Work out the finished part from the listing and answer in its coordinate system (mm). A direction names the side the tool comes from. Round coordinates to 2 decimals unless told otherwise and drop trailing zeros. Loops run counter-clockwise (first coordinate to the right, second up) from the corner with the lowest first, then second, coordinate; pieces in that order, holes last.
from build123d import *

# Parameters (mm, degrees)
SKETCH_1_W           = 149
SKETCH_1_H           = 70
EXTRUDE_1_DEPTH      = 1
SKETCH_2_W           = 147
SKETCH_2_H           = 68
EXTRUDE_2_DEPTH      = 2
FILLET_1_R           = 5
SKETCH_3_W           = 3
SKETCH_3_H           = 26
EXTRUDE_3_DEPTH      = 10
FILLET_2_R           = 4
SKETCH_6_R           = 3.5
EXTRUDE_4_DEPTH      = 4
SKETCH_7_W           = 86.66
SKETCH_7_H           = 55.5
CUT_EXTRUDE_3_DEPTH  = 2
SKETCH_8_W           = 74
SKETCH_8_H           = 49
CUT_EXTRUDE_4_DEPTH  = 2
SKETCH_11_R          = 4
CUT_EXTRUDE_7_DEPTH  = 4
SKETCH_12_R          = 1.35
CUT_EXTRUDE_8_DEPTH  = 4
SKETCH_13_R          = 1.35
CUT_EXTRUDE_9_DEPTH  = 4
SKETCH_14_R          = 1.35
CUT_EXTRUDE_10_DEPTH = 4
SKETCH_15_W          = 14
SKETCH_15_H          = 13.5
CUT_EXTRUDE_11_DEPTH = 4
SKETCH_9_R           = 3.5
CUT_EXTRUDE_12_DEPTH = 4
SKETCH_16_R          = 3.5
CUT_EXTRUDE_13_DEPTH = 4
EXTRUDE_5_DEPTH      = 4
EXTRUDE_6_DEPTH      = 1


with BuildPart() as part:
    # Эскиз1 → Бобышка-Вытянуть1 (new body)
    with BuildSketch(Plane.XY):
        Rectangle(SKETCH_1_W, SKETCH_1_H)
    extrude(amount=EXTRUDE_1_DEPTH)

    # Эскиз2 → Бобышка-Вытянуть2 (add)
    with BuildSketch(Plane.XY.offset(1)):
        Rectangle(SKETCH_2_W, SKETCH_2_H)
    extrude(amount=EXTRUDE_2_DEPTH)

    # Скругление1
    fillet_1_edges = [part.edges().sort_by_distance(p)[0] for p in [
        (-73.5, 34, 2),
        (-73.5, -34, 2),
        (73.5, -34, 2),
        (73.5, 34, 2),
        (-74.5, 35, 0.5),
        (74.5, 35, 0.5),
        (74.5, -35, 0.5),
        (-74.5, -35, 0.5),
    ]]
    fillet(fillet_1_edges, radius=FILLET_1_R)

    # Эскиз3 → Бобышка-Вытянуть3 (add)
    with BuildSketch(Plane.XY.offset(3)):
        with Locations((-72, 1)):
            Rectangle(SKETCH_3_W, SKETCH_3_H)
        with Locations((72, 1)):
            Rectangle(SKETCH_3_W, SKETCH_3_H)
    extrude(amount=EXTRUDE_3_DEPTH)

    # Скругление2
    fillet_2_edges = [part.edges().sort_by_distance(p)[0] for p in [
        (-72, -12, 13),
        (-72, 14, 13),
        (72, 14, 13),
        (72, -12, 13),
    ]]
    fillet(fillet_2_edges, radius=FILLET_2_R)

    # Эскиз6 → Бобышка-Вытянуть4 (add)
    with BuildSketch(Plane.XY.offset(3)):
        with Locations((-67.16, 29.285)):
            Circle(SKETCH_6_R)
        with Locations((67.16, 29.285)):
            Circle(SKETCH_6_R)
        with Locations((-67.16, -29.285)):
            Circle(SKETCH_6_R)
    extrude(amount=EXTRUDE_4_DEPTH)

    # Эскиз7 → Вырез-Вытянуть3 (cut)
    with BuildSketch(Plane.XY.offset(3)):
        with Locations((12.83, 4.75)):
            Rectangle(SKETCH_7_W, SKETCH_7_H)
    extrude(amount=-CUT_EXTRUDE_3_DEPTH, mode=Mode.SUBTRACT)

    # Эскиз8 → Вырез-Вытянуть4 (cut, through all)
    with BuildSketch(Plane.XY.offset(1)):
        with Locations((15.66, 4.3)):
            Rectangle(SKETCH_8_W, SKETCH_8_H)
    extrude(amount=-CUT_EXTRUDE_4_DEPTH, mode=Mode.SUBTRACT)

    # Эскиз11 → Вырез-Вытянуть7 (cut, through all)
    with BuildSketch(Plane.XY.offset(3)):
        with Locations((-53.163, 18.448)):
            Circle(SKETCH_11_R)
        with Locations((-53.163, -12.552)):
            Circle(SKETCH_11_R)
    extrude(amount=-CUT_EXTRUDE_7_DEPTH, mode=Mode.SUBTRACT)

    # Эскиз12 → Вырез-Вытянуть8 (cut)
    with BuildSketch(Plane.XY.offset(7)):
        with Locations((-67.16, 29.285)):
            Circle(SKETCH_12_R)
    extrude(amount=-CUT_EXTRUDE_8_DEPTH, mode=Mode.SUBTRACT)

    # Эскиз13 → Вырез-Вытянуть9 (cut)
    with BuildSketch(Plane.XY.offset(7)):
        with Locations((67.16, 29.285)):
            Circle(SKETCH_13_R)
    extrude(amount=-CUT_EXTRUDE_9_DEPTH, mode=Mode.SUBTRACT)

    # Эскиз14 → Вырез-Вытянуть10 (cut)
    with BuildSketch(Plane.XY.offset(7)):
        with Locations((-67.16, -29.285)):
            Circle(SKETCH_14_R)
    extrude(amount=-CUT_EXTRUDE_10_DEPTH, mode=Mode.SUBTRACT)

    # Эскиз15 → Вырез-Вытянуть11 (cut, through all)
    with BuildSketch(Plane.XY.offset(3)):
        with Locations((65, -20.05)):
            Rectangle(SKETCH_15_W, SKETCH_15_H)
    extrude(amount=-CUT_EXTRUDE_11_DEPTH, mode=Mode.SUBTRACT)

    # Эскиз9 → Вырез-Вытянуть12 (cut, through all)
    with BuildSketch(Plane.XY.offset(3)):
        with Locations((62.54, -6.405)):
            Circle(SKETCH_9_R)
        with Locations((62.54, 21.595)):
            Circle(SKETCH_9_R)
        with Locations((62.54, 7.595)):
            Circle(SKETCH_9_R)
    extrude(amount=-CUT_EXTRUDE_12_DEPTH, mode=Mode.SUBTRACT)

    # Эскиз16 → Вырез-Вытянуть13 (cut, through all)
    with BuildSketch(Plane.XY.offset(3)):
        with Locations((45.24, -27.88)):
            Circle(SKETCH_16_R)
        with Locations((29.49, -27.88)):
            Circle(SKETCH_16_R)
        with Locations((13.47, -27.88)):
            Circle(SKETCH_16_R)
        with Locations((-2.28, -27.88)):
            Circle(SKETCH_16_R)
        with Locations((-18.03, -27.88)):
            Circle(SKETCH_16_R)
        with Locations((-33.78, -27.88)):
            Circle(SKETCH_16_R)
    extrude(amount=-CUT_EXTRUDE_13_DEPTH, mode=Mode.SUBTRACT)

    # Эскиз17 → Бобышка-Вытянуть5 (add)
    with BuildSketch(Plane.XY.offset(3)):
        with BuildLine():
            Line((68.5, -34), (-68.5, -34))
            ThreePointArc((-68.5, -34), (-72.035533906, -32.535533906), (-73.5, -29))
            Line((-73.5, -29), (-73.5, 29))
            ThreePointArc((-73.5, 29), (-72.035533906, 32.535533906), (-68.5, 34))
            Line((-68.5, 34), (68.5, 34))
            ThreePointArc((68.5, 34), (72.035533906, 32.535533906), (73.5, 29))
            Line((73.5, 29), (73.5, -29))
            ThreePointArc((73.5, -29), (72.035533906, -32.535533906), (68.5, -34))
        make_face()
        with BuildLine():
            Line((67, -32.5), (-67, -32.5))
            ThreePointArc((-67, -32.5), (-70.535533906, -31.035533906), (-72, -27.5))
            Line((-72, -27.5), (-72, 27.5))
            ThreePointArc((-72, 27.5), (-70.535533906, 31.035533906), (-67, 32.5))
            Line((-67, 32.5), (67, 32.5))
            ThreePointArc((67, 32.5), (70.535533906, 31.035533906), (72, 27.5))
            Line((72, 27.5), (72, -27.5))
            ThreePointArc((72, -27.5), (70.535533906, -31.035533906), (67, -32.5))
        make_face(mode=Mode.SUBTRACT)
    extrude(amount=EXTRUDE_5_DEPTH)

    # Эскиз18 → Бобышка-Вытянуть6 (add)
    with BuildSketch(Plane.XY.offset(1)):
        with BuildLine():
            Line((69.5, -35), (-69.5, -35))
            ThreePointArc((-69.5, -35), (-73.035533906, -33.535533906), (-74.5, -30))
            Line((-74.5, -30), (-74.5, 30))
            ThreePointArc((-74.5, 30), (-73.035533906, 33.535533906), (-69.5, 35))
            Line((-69.5, 35), (69.5, 35))
            ThreePointArc((69.5, 35), (73.035533906, 33.535533906), (74.5, 30))
            Line((74.5, 30), (74.5, -30))
            ThreePointArc((74.5, -30), (73.035533906, -33.535533906), (69.5, -35))
        make_face()
        with BuildLine():
            Line((68.5, -34), (-68.5, -34))
            ThreePointArc((-68.5, -34), (-72.035533906, -32.535533906), (-73.5, -29))
            Line((-73.5, -29), (-73.5, 29))
            ThreePointArc((-73.5, 29), (-72.035533906, 32.535533906), (-68.5, 34))
            Line((-68.5, 34), (68.5, 34))
            ThreePointArc((68.5, 34), (72.035533906, 32.535533906), (73.5, 29))
            Line((73.5, 29), (73.5, -29))
            ThreePointArc((73.5, -29), (72.035533906, -32.535533906), (68.5, -34))
        make_face(mode=Mode.SUBTRACT)
    extrude(amount=EXTRUDE_6_DEPTH)


solid = part.part
Item 1: Section D-D, the plane x = -33.78 is taken. Give the vertices of the cut face in (y, z), plus the area to 3 significant figures.
Item 2: Each of these flat-tipped pins is pushed along its axis until it touches: P1, Ø11, axis at x = 22.5, y = -22.5, coming from the +Z side; P2, Ø3, axis at y = -1.5, z = 8, coming from the -X side; P3, Ø4.5, axis at y = -19, z = 4.5, coming from the +X side. Where does it stop, or does it pass through?
Item 3: Section A-A, the plane x = 22 is taken. Give the vertices of the cut face in (y, z).
Item 4: For faces 1 (the face through (-0.4, -24.93, 1.52)), 2 (the face through (-73.5, 0, 6)), 3 (the face through (67, 29, 3)), determine the directions among +Z, -Z, +X, -X, +Y, -Y from which every point of the face is accessible in a straight line to the end or side of a thin tool.
Item 5: Straight lines are drawn through the part: line 1 (Y direction, x = -18.03, z = 1.6); line 2 (Y direction, x = 62.54, z = 1.7) (3 decimals); line 3 (X direction, y = 19, z = 5.5). For each, find the intervals that lie inside material, in ascending order.
Item 6: Determine the mould class of faces 4 (the face through (-1, 34, 4)), 5 (the face through (29.03, -24.41, 1.52)), 6 (the face through (-71.979, -10.859, 11.797)), 7 (the face through (0, 33, 7)) for opening direction Y: pulls with the +Y half, pulls with the -Y half, needs draft (parallel to the pull), parting line crosses it, or undercut.
Item 7: Section C-C, the plane z = 5.5 is taken. State how many separate pieces and enclosed holes the cut face has, plus the area to 3 significant figures.
Item 8: Section B-B, the plane x = -18.03 is taken. Give the vertices of the cut face in (y, z).
Answer below:
1. outline: (-35, 0) - (-31.38, 0) - (-31.38, 3) - (-32.5, 3) - (-32.5, 7) - (-34, 7) - (-34, 2) - (-35, 2) - close; (-24.38, 0) - (35, 0) - (35, 2) - (34, 2) - (34, 7) - (32.5, 7) - (32.5, 3) - (-24.38, 3) - close
1. area: 199 mm2
2. P1: stops at z = 3
2. P2: stops at x = -73.5
2. P3: stops at x = 73.5
3. outline: (-35, 0) - (-20.2, 0) - (-20.2, 1) - (-23, 1) - (-23, 3) - (-32.5, 3) - (-32.5, 7) - (-34, 7) - (-34, 2) - (-35, 2) - close; (28.8, 0) - (35, 0) - (35, 2) - (34, 2) - (34, 7) - (32.5, 7) - (32.5, 1) - (28.8, 1) - close
4. face 1: +Z, -Z
4. face 2: +Z, -X, +Y, -Y
4. face 3: +Z
5. line 1: y = -35 to -31.38, -24.38 to -23, 32.5 to 35
5. line 2: y = -35 to -26.8, -13.3 to -9.905, -2.905 to 4.095, 11.095 to 18.095, 25.095 to 35
5. line 3: x = -73.5 to -72, 72 to 73.5
6. face 4: pulls with the +Y half
6. face 5: undercut
6. face 6: pulls with the -Y half
6. face 7: needs draft
7. separate pieces: 1
7. enclosed holes: 4
7. area: 810 mm2
8. outline: (-35, 0) - (-31.38, 0) - (-31.38, 3) - (-32.5, 3) - (-32.5, 7) - (-34, 7) - (-34, 2) - (-35, 2) - close; (-24.38, 0) - (-20.2, 0) - (-20.2, 1) - (-23, 1) - (-23, 3) - (-24.38, 3) - close; (28.8, 0) - (35, 0) - (35, 2) - (34, 2) - (34, 7) - (32.5, 7) - (32.5, 1) - (28.8, 1) - close
